Autodesk Fusion 360 part; units mm, degrees
sketch "Sketch1" plane through (0, 0, -20.5) normal (0, 0, -1) x (-1, 0, 0)
  line L0 (-5, 0) -> (-5, -15)
  line L1 (-5, -15) -> (70, -15)
  line L2 (70, -15) -> (70, 0)
  circle A0 centre (0, -10.5) radius 1
  circle A1 centre (21, -10.5) radius 1
  circle A2 centre (0, 0) radius 7.0711
  line L3 (67, -10.3624) -> (65, -10.3624)
  line L4 (65, -10.3624) -> (65, -2.8871)
  line L5 (65, -2.8871) -> (67, -2.8871)
  line L6 (67, -2.8871) -> (67, -10.3624)
  line L7 (100, 0) -> (42, 0) construction
  line L8 (-5, 15) -> (70, 15)
  line L9 (70, 15) -> (70, 0)
  line L10 (67, 10.3624) -> (65, 10.3624)
  line L11 (67, 2.8871) -> (67, 10.3624)
  line L12 (65, 10.3624) -> (65, 2.8871)
  line L13 (65, 2.8871) -> (67, 2.8871)
  circle A3 centre (21, 10.5) radius 1
  circle A4 centre (0, 10.5) radius 1
  line L14 (-5, 0) -> (-5, 15)
  line L15 (27.9727, 11.0949) -> (37.9727, 11.0949)
  line L16 (37.9727, 11.0949) -> (37.9727, 9.0949)
  line L17 (37.9727, 9.0949) -> (27.9727, 9.0949)
  line L18 (27.9727, 9.0949) -> (27.9727, 11.0949)
  line L19 (42.9727, 11.2127) -> (42.9727, -12.2873) construction
  line L20 (42.9727, -11.2127) -> (42.9727, 12.2873) construction
  line L21 (37.9727, -11.0949) -> (37.9727, -9.0949)
  line L22 (37.9727, -9.0949) -> (27.9727, -9.0949)
  line L23 (27.9727, -9.0949) -> (27.9727, -11.0949)
  line L24 (27.9727, -11.0949) -> (37.9727, -11.0949)
  line L25 (57.9727, 11.0949) -> (47.9727, 11.0949)
  line L26 (47.9727, 11.0949) -> (47.9727, 9.0949)
  line L27 (47.9727, 9.0949) -> (57.9727, 9.0949)
  line L28 (57.9727, 9.0949) -> (57.9727, 11.0949)
  line L29 (47.9727, -11.0949) -> (47.9727, -9.0949)
  line L30 (57.9727, -9.0949) -> (57.9727, -11.0949)
  line L31 (47.9727, -9.0949) -> (57.9727, -9.0949)
  line L32 (57.9727, -11.0949) -> (47.9727, -11.0949)
  dimension "d1" = 75
  dimension "d3" = 2
  dimension "d4" = 3
  dimension "d77" = 0
  dimension "d78" = 0
  dimension "d79" = 0
  dimension "d80" = 0
  dimension "d93" = 10
  dimension "d94" = 2
  dimension "d95" = 10
extrude "Extrude1" add sketch "Sketch1" along normal blind 2 contours L0 L1 L2 A2 L8 L9 L14
sketch "Sketch2" plane through (0, 0, -22.5) normal (0, 0, -1) x (-1, 0, 0)
  line L0 (25, -6.0704) -> (55, -6.0704)
  arc A0 (55, -6.0704) -> (55, 6.0704) centre (55, 0) ccw
  line L1 (55, 6.0704) -> (25, 6.0704)
  arc A1 (25, 6.0704) -> (25, -6.0704) centre (25, 0) ccw
  line L2 (25, 0) -> (55, 0) construction
  line L3 (100, 0) -> (42, 0)
extrude "Extrude2" cut sketch "Sketch2" against normal blind 2
fillet "Fillet1" radius 3 6 edges at (5, 15, -21.5) (5, 5, -21.5) (5, -5, -21.5) (5, -15, -21.5) (-70, 15, -21.5) (-70, -15, -21.5)
sketch "Sketch3" plane through (0, 0, -20.5) normal (0, 0, 1) x (1, 0, 0)
sketch "projection" plane through (0, 0, -20.5) normal (0, 0, 1) x (1, 0, 0)
  line L0 (-25, -6.0704) -> (-55, -6.0704)
  arc A0 (-55, 6.0704) -> (-55, -6.0704) centre (-55, 0) ccw
  line L1 (-55, 6.0704) -> (-25, 6.0704)
  arc A1 (-25, -6.0704) -> (-25, 6.0704) centre (-25, 0) ccw
  circle A2 centre (-21, 10.5) radius 1
  line L2 (-57.9727, -11.0949) -> (-57.9727, -9.0949)
  line L3 (-57.9727, -9.0949) -> (-47.9727, -9.0949)
  line L4 (-47.9727, -9.0949) -> (-47.9727, -11.0949)
  line L5 (-47.9727, -11.0949) -> (-57.9727, -11.0949)
  circle A3 centre (0, 10.5) radius 1
  line L6 (-65, 2.8871) -> (-67, 2.8871)
  line L7 (-67, 2.8871) -> (-67, 10.3624)
  line L8 (-67, 10.3624) -> (-65, 10.3624)
  line L9 (-65, 10.3624) -> (-65, 2.8871)
  line L10 (-27.9727, -11.0949) -> (-37.9727, -11.0949)
  line L11 (-37.9727, -11.0949) -> (-37.9727, -9.0949)
  line L12 (-37.9727, -9.0949) -> (-27.9727, -9.0949)
  line L13 (-27.9727, -9.0949) -> (-27.9727, -11.0949)
  circle A4 centre (0, -10.5) radius 1
  line L14 (-57.9727, 9.0949) -> (-57.9727, 11.0949)
  line L15 (-57.9727, 11.0949) -> (-47.9727, 11.0949)
  line L16 (-47.9727, 11.0949) -> (-47.9727, 9.0949)
  line L17 (-47.9727, 9.0949) -> (-57.9727, 9.0949)
  circle A5 centre (-21, -10.5) radius 1
  line L18 (-67, -2.8871) -> (-65, -2.8871)
  line L19 (-65, -2.8871) -> (-65, -10.3624)
  line L20 (-65, -10.3624) -> (-67, -10.3624)
  line L21 (-67, -10.3624) -> (-67, -2.8871)
  line L22 (-27.9727, 9.0949) -> (-37.9727, 9.0949)
  line L23 (-37.9727, 9.0949) -> (-37.9727, 11.0949)
  line L24 (-37.9727, 11.0949) -> (-27.9727, 11.0949)
  line L25 (-27.9727, 11.0949) -> (-27.9727, 9.0949)
  arc A6 (-70, -12) -> (-67, -15) centre (-67, -12) ccw
  line L26 (-67, -15) -> (2, -15)
  arc A7 (2, -15) -> (5, -12) centre (2, -12) ccw
  line L27 (5, -12) -> (5, -9.8705)
  arc A8 (5, -9.8705) -> (1.4042, -6.9302) centre (2, -9.8705) ccw
  arc A9 (1.4042, 6.9302) -> (1.4042, -6.9302) centre (0, 0) ccw
  arc A10 (1.4042, 6.9302) -> (5, 9.8705) centre (2, 9.8705) ccw
  line L28 (5, 9.8705) -> (5, 12)
  arc A11 (5, 12) -> (2, 15) centre (2, 12) ccw
  line L29 (2, 15) -> (-67, 15)
  arc A12 (-67, 15) -> (-70, 12) centre (-67, 12) ccw
  line L30 (-70, 12) -> (-70, -12)
equation "thiccness = 2 mm"
equation "d3 = thiccness"
equation "d11 = thiccness"
equation "d94 = thiccness"
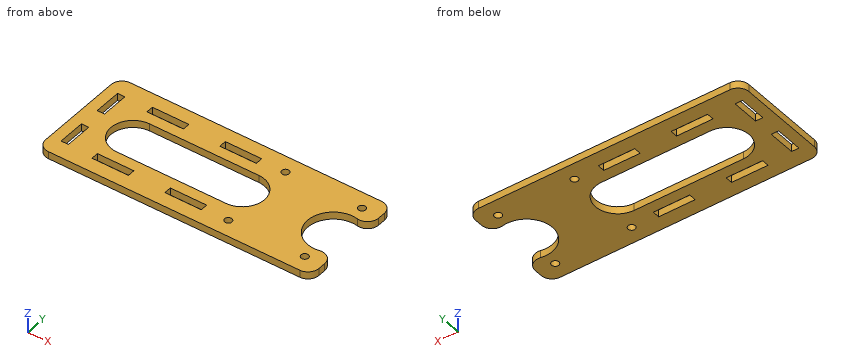
The listing builds one solid part. Answer for the finished solid, in the listing's coordinates (mm). Coordinates: 2 decimals unless noted, no trailing zeros. Loops run counter-clockwise (first coordinate to the right, second up) from the corner with the lowest first, then second, coordinate; pieces in that order, holes last. Notation, with made-up numbers: (26.25, 76) -> (48.25, 76) arc R29 ccw to (48.25, 113) -> close; hole circle Ø2 at (14, 37.5). An arc over 180 degrees is marked (long way). Write item = value, one per line. Start each with the question number.
1) A cutting plane is placed at A-A (y = 0). Give the vertices of the cut face in (x, z), then the cut area to 3 significant figures.
2) Given pin 1 Ø1 at (y, z) = (-8, -21.5) entering from +X; pin 2 Ø1.6 at (x, y) = (0, -10.5) entering from +Z, each flat-ended and moving along its own axis, determine where each tip first touches the part or whether it passes through.
3) A cutting plane is placed at B-B (x = -57). Give the vertices of the cut face in (y, z), then the cut area to 3 significant figures.
4) A cutting plane is placed at D-D (z = -21.65). Count the separate pieces of the cut face and the enclosed holes in it, then the cut area to 3 significant figures.
5) A cutting plane is placed at C-C (x = 0). Give the vertices of the cut face in (y, z).
6) Straight lines are drawn through the part: line 1 (Y direction, x = 2, z = -21.65); line 2 (X direction, y = 0, z = -21.7); line 3 (Y direction, x = -24.5, z = -22.1). For each, find the intervals that lie inside material, in ascending order. Write a range as from..to.
Responses:
q1.outline = (-70, -22.5) -> (-61.07, -22.5) -> (-61.07, -20.5) -> (-70, -20.5) -> close; (-18.93, -22.5) -> (-7.07, -22.5) -> (-7.07, -20.5) -> (-18.93, -20.5) -> close
q1.area = 41.6 mm²
q2.pin_1 = 4.67
q2.pin_2 = through
q3.outline = (-15, -22.5) -> (-11.09, -22.5) -> (-11.09, -20.5) -> (-15, -20.5) -> close; (-9.09, -22.5) -> (-5.73, -22.5) -> (-5.73, -20.5) -> (-9.09, -20.5) -> close; (5.73, -22.5) -> (9.09, -22.5) -> (9.09, -20.5) -> (5.73, -20.5) -> close; (11.09, -22.5) -> (15, -22.5) -> (15, -20.5) -> (11.09, -20.5) -> close
q3.area = 29.1 mm²
q4.separate_pieces = 1
q4.enclosed_holes = 11
q4.area = 1,490 mm²
q5.outline = (-15, -22.5) -> (-11.5, -22.5) -> (-11.5, -20.5) -> (-15, -20.5) -> close; (-9.5, -22.5) -> (-7.07, -22.5) -> (-7.07, -20.5) -> (-9.5, -20.5) -> close; (7.07, -22.5) -> (9.5, -22.5) -> (9.5, -20.5) -> (7.07, -20.5) -> close; (11.5, -22.5) -> (15, -22.5) -> (15, -20.5) -> (11.5, -20.5) -> close
q6.line_1 = -15..-6.87, 6.87..15
q6.line_2 = -70..-61.07, -18.93..-7.07
q6.line_3 = -15..-6.05, 6.05..15
